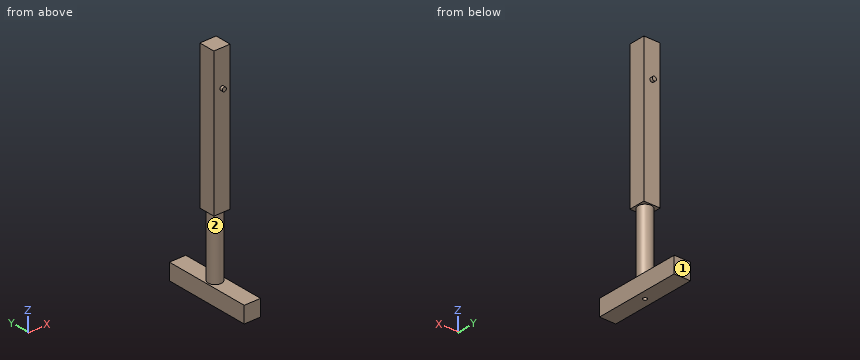
```python
from build123d import *

# Parameters (mm, degrees)
SKETCH_1_W          = 60
SKETCH_1_H          = 60
EXTRUDE_1_DEPTH     = 530
SKETCH_2_R          = 25
EXTRUDE_2_DEPTH     = 230
SKETCH_3_R          = 7.5
EXTRUDE_3_DEPTH     = 10
EXTRUDE_START       = 10
SKETCH_4_R          = 7.5
EXTRUDE_4_DEPTH     = 10
SKETCH_5_W          = 60
SKETCH_5_H          = 320
EXTRUDE_5_DEPTH     = 60
SKETCH_6_R          = 7.5
CUT_EXTRUDE_1_DEPTH = 40


with BuildPart() as part:
    # 草图1 → 凸台-拉伸1 (new body)
    with BuildSketch(Plane.XY):
        Rectangle(SKETCH_1_W, SKETCH_1_H)
    extrude(amount=EXTRUDE_1_DEPTH)

    # 草图2 → 凸台-拉伸2 (add)
    with BuildSketch(Plane(origin=(0, 0, 0), x_dir=(-1, 0, 0), z_dir=(0, 0, -1))):
        Circle(SKETCH_2_R)
    extrude(amount=EXTRUDE_2_DEPTH)

    # 草图3 → 凸台-拉伸3 (add)
    with BuildSketch(Plane(origin=(0, 30, 0), x_dir=(1, 0, 0), z_dir=(0, 1, 0))):
        with Locations(Location((0, -400, 0), (0, 0, 90))):
            Circle(SKETCH_3_R)
    extrude(amount=EXTRUDE_3_DEPTH)

    # 草图4 → 凸台-拉伸4 (add)
    with BuildSketch(Plane.XZ.offset(30).offset(EXTRUDE_START)):
        with Locations(Location((0, 400, 0), (0, 0, 270))):
            Circle(SKETCH_4_R)
    extrude(amount=-EXTRUDE_4_DEPTH)

    # 草图5 → 凸台-拉伸5 (add)
    with BuildSketch(Plane(origin=(0, 0, -230), x_dir=(-1, 0, 0), z_dir=(0, 0, -1))):
        Rectangle(SKETCH_5_W, SKETCH_5_H)
    extrude(amount=EXTRUDE_5_DEPTH)

    # 草图6 → 切除-拉伸1 (cut)
    with BuildSketch(Plane(origin=(0, 0, -290), x_dir=(-1, 0, 0), z_dir=(0, 0, -1))):
        Circle(SKETCH_6_R)
    extrude(amount=-CUT_EXTRUDE_1_DEPTH, mode=Mode.SUBTRACT)


solid = part.part
```
Verification items for the finished model (mm, model axes). Face numbers are marked on the shaded views. Give positions to 0.01 mm unless a question says otherwise; leave off trailing zeros. Order: outer loops, then holes, each group sorted by start corner. A loop starts at its lowest first (then second) coordinate and runs counter-clockwise, first axis right, second up. Notation, with made-up numbers: M 15,-38.75 L 39,-38.75 A23 ccw 39,-18.75 Z; hole C 82,29.25 d3. An arc over 180 degrees is marked long. Return JSON: item names as keys, results as strings. Group by question number.
1) Section check B-B on z = 400. Record the cut outline in (x, y).
2) Section check A-A on x = 0. Record the cut outline in (y, z).
3) Section check C-C on y = 0. Record the cut outline in (x, z).
4) Section check D-D on y = 114.5. Record the cut outline in (x, z), and give its area (3 significant figures).
5) Mould release check, pull along Z, two halves, no side actions. Record for the marked faces 1 and 2: pulls with the +Z half, pulls with the -Z half, needs draft (parallel to the pull), parting line crosses it, or undercut.
6) Scan lines: line 1 (Y direction, x = 0, z = -264.5); line 2 (Z direction, x = 25, y = -33.5); line 3 (Y direction, x = -24.5, z = 477). Record each from-to range of solid material in increasing order.
7) Go/stop test with flat-tipped pins: pin 1 Ø16.5 at (x, z) = (-2, 402.5) entering from +Y; pin 2 Ø3 at (y, z) = (17, -24.5) entering from +X; pin 3 Ø10 at (x, y) = (-22, 41.5) entering from +Z. Record where each tip stops, or that it passes through.
Answer block:
{
 "1": {"outline": "M -30,-30 L -7.5,-30 L -7.5,-40 L 7.5,-40 L 7.5,-30 L 30,-30 L 30,30 L 7.5,30 L 7.5,40 L -7.5,40 L -7.5,30 L -30,30 Z"},
 "2": {"outline": "M -160,-290 L -7.5,-290 L -7.5,-250 L 7.5,-250 L 7.5,-290 L 160,-290 L 160,-230 L 25,-230 L 25,0 L 30,0 L 30,392.5 L 40,392.5 L 40,407.5 L 30,407.5 L 30,530 L -30,530 L -30,407.5 L -40,407.5 L -40,392.5 L -30,392.5 L -30,0 L -25,0 L -25,-230 L -160,-230 Z"},
 "3": {"outline": "M -30,-290 L -7.5,-290 L -7.5,-250 L 7.5,-250 L 7.5,-290 L 30,-290 L 30,-230 L 25,-230 L 25,0 L 30,0 L 30,530 L -30,530 L -30,0 L -25,0 L -25,-230 L -30,-230 Z"},
 "4": {"outline": "M -30,-290 L 30,-290 L 30,-230 L -30,-230 Z", "area": "3,600 mm^2"},
 "5": {"face 1": "needs draft", "face 2": "undercut"},
 "6": {"line 1": "y = -160 to -7.5, 7.5 to 160", "line 2": "z = -290 to -230", "line 3": "y = -30 to 30"},
 "7": {"pin 1": "stops at y = 40", "pin 2": "stops at x = 19.62", "pin 3": "stops at z = -230"}
}
